```python
from build123d import *

# Parameters (mm, degrees)
F1_DEPTH = 12.7


with BuildPart() as f1:
    # F0 (on Top) → F1 (new body)
    with BuildSketch(Plane.XY):
        with BuildLine():
            ThreePointArc((0, 16.66875), (11.786586, 11.786586), (16.66875, 0))
            Line((16.66875, 0), (16.66875, -12.065))
            ThreePointArc((16.66875, -12.065), (17.784673, -14.759077), (20.47875, -15.875))
            Line((20.47875, -15.875), (35.71875, -15.875))
            Line((35.71875, -15.875), (35.71875, -12.293821))
            Line((35.71875, -12.293821), (26.822409, -12.293821))
            add(Edge.make_bspline(
                [(19.05, 0), (19.807434, -4.250921), (16.66875, -12.065), (26.822409, -12.293821)],
                knots=[0, 0, 0, 0, 14.544702, 14.544702, 14.544702, 14.544702], degree=3))
            ThreePointArc((19.05, 0), (13.470384, 13.470384), (0, 19.05))
            ThreePointArc((0, 19.05), (-13.470384, 13.470384), (-19.05, 0))
            add(Edge.make_bspline(
                [(-19.05, 0), (-19.807434, -4.250921), (-16.66875, -12.065), (-26.822409, -12.293821)],
                knots=[0, 0, 0, 0, 14.544702, 14.544702, 14.544702, 14.544702], degree=3))
            Line((-26.822409, -12.293821), (-35.71875, -12.293821))
            Line((-35.71875, -12.293821), (-35.71875, -15.875))
            Line((-35.71875, -15.875), (-20.47875, -15.875))
            ThreePointArc((-20.47875, -15.875), (-17.784673, -14.759077), (-16.66875, -12.065))
            Line((-16.66875, -12.065), (-16.66875, 0))
            ThreePointArc((-16.66875, 0), (-11.786586, 11.786586), (0, 16.66875))
        make_face()
    extrude(amount=F1_DEPTH)


solid = f1.part
```
Model file for the job. Use its own axes, mm. A direction names the side the tool comes from. Coordinates: 2 decimals unless noted, no trailing zeros. Write each loop counter-clockwise with the first axis right and the second up, starting at its lowest first coordinate (ties: lowest second). Pieces come first, ordered by that corner, then holes. Notation, with made-up numbers: (41.25, -12.5) - (66.25, -12.5) arc R36 ccw to (66.25, 21.5) - close; hole circle Ø3 at (8.25, -25). An arc over 180 degrees is marked (long way). One line per question, with ' | ' between items. Start each with the question number.
Q1. 3-axis set-ups, long thin cutter, end or side, ignore diameter. For faces 5 (the face through (-16, 6, 0)), 6 (the face through (-31, -12.294, 6)), 7 (the face through (31, -12.294, 6)), 8 (the face through (-16.669, -6, 6)): which of +Z, -Z, +X, -X, +Y, -Y reach the whole face in a straight line?
Q2. Cut at D-D, the plane x = -18. List the corners of the cut face in (y, z), then the cut area to 3 significant figures.
Q3. Cut at A-A, the plane y = 1. List the corners of the cut face in (x, z), then the cut area to 3 significant figures.
Q4. Pull direction X, two halves, no side cores. Call faces 1 (the face through (16.669, -6, 6)), 2 (the face through (35.719, -14, 6)), 3 (the face through (-16, 6, 12.7)), 4 (the face through (-35.719, -14, 6)): pulls with the +X half, pulls with the -X half, needs draft (parallel to the pull), parting line crosses it, or undercut.
Q5. Cut at C-C, the plane x = 30.5. List the corners of the cut face in (y, z) (3 decimals), then the cut area to 3 significant figures.
Q6. Drill centre lines: line 1 (X direction, y = 0.5, z = 12); line 2 (Y direction, x = 26.5, z = 4.5) (3 decimals); line 3 (X direction, y = 12.5, z = 5.25). Where is each one in solid material? Low to high. Write a range as [from, to].
Q7. Pin check, flat tips, straight feed: pin 1 (4.5 mm diameter, centred on x = -31.5, z = 3, fed in from +Y); pin 2 (2 mm diameter, centred on x = 6.5, z = 9, fed in from +Y); pin 3 (6 mm diameter, centred on y = 11, z = 5, fed in from +X). Stop position of each tip, or through.
Q8. Cut at B-B, the plane y = 14.5. List the corners of the cut face in (x, z), then the cut area to 3 significant figures.
Answer below:
1) face 5: -Z, +X, -X, +Y, -Y | face 6: +Z, -Z, -X, +Y | face 7: +Z, -Z, +X, +Y | face 8: +Z, -Z, -Y
2) outline: (-14.96, 0) - (6.24, 0) - (6.24, 12.7) - (-14.96, 12.7) - close | area: 269 mm^2
3) outline: (-19.02, 0) - (-16.64, 0) - (-16.64, 12.7) - (-19.02, 12.7) - close; (16.64, 0) - (19.02, 0) - (19.02, 12.7) - (16.64, 12.7) - close | area: 60.6 mm^2
4) face 1: undercut | face 2: pulls with the +X half | face 3: needs draft | face 4: pulls with the -X half
5) outline: (-15.875, 0) - (-12.294, 0) - (-12.294, 12.7) - (-15.875, 12.7) - close | area: 45.5 mm^2
6) line 1: [-19.04, -16.66], [16.66, 19.04] | line 2: [-15.875, -12.284] | line 3: [-14.38, -11.03], [11.03, 14.38]
7) pin 1: y = -12.29 | pin 2: y = 18.24 | pin 3: x = 17.29
8) outline: (-12.36, 0) - (-8.22, 0) - (-8.22, 12.7) - (-12.36, 12.7) - close; (8.22, 0) - (12.36, 0) - (12.36, 12.7) - (8.22, 12.7) - close | area: 105 mm^2
